For this review, take the finished solid that the model builds, in its own axes (mm). Face numbers are marked on the shaded views. Coordinates: 2 decimals unless noted, no trailing zeros. Loops run counter-clockwise (first coordinate to the right, second up) from the corner with the lowest first, then second, coordinate; pieces in that order, holes last. Notation, with made-up numbers: (-33, -35) - (23, -35) arc R13 cw to (23, -12) - close; hole circle Ø1 at (72.25, 76). An arc over 180 degrees is marked (long way). Use one line per item in the form item = value. Start each with the question number.
1. Add section C-C on z = 41. Give the boundary of the cut face in (x, y).
2. To check wall thickness, follow probe 1 along Y at (x, z) = (0, 23.25); probe 2 along Y at (x, z) = (0, 0.25); probe 3 along Z at (x, y) = (-8.5, -10.5). State the ranges of each line that lie inside material, in increasing order.
3. Add section A-A on z = 20.5. Give the boundary of the cut face in (x, y).
4. For pin 1 Ø1 at (x, z) = (3.5, 31.5) entering from +Y; pin 2 Ø2 at (x, z) = (-3.5, 41) entering from +Y; pin 3 Ø3 at (y, z) = (15, 38.5) entering from +X, all flat-tipped, find the tip position at first contact; note any pin that passes through.
5. Add section D-D on y = -11.25. Give the boundary of the cut face in (x, z).
6. Draft analysis for pull direction Y (two halves, no side actions). For the marked faces 1, 2 and 3, state which applies: +Y half, -Y half, draft (parallel to the pull), parting line (faces both ways), or undercut.
7. Add section B-B on x = 0. Give the boundary of the cut face in (y, z).
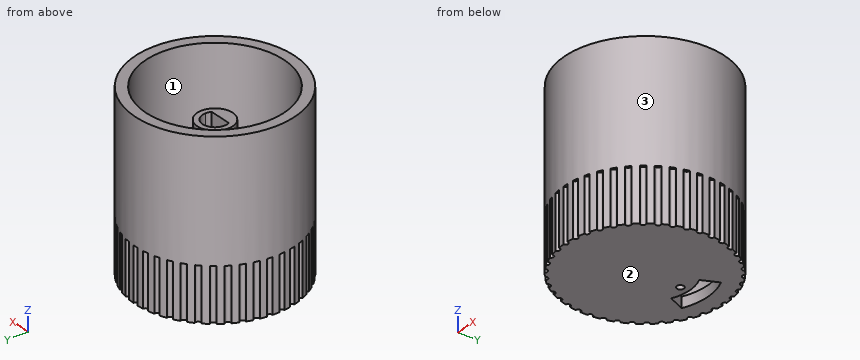
```python
from build123d import *

# Parameters (mm, degrees)
F10_R     = 22.5
F0_DEPTH  = 48.6
F1_T      = -3
F2_R      = 5
F3_DEPTH  = 37
F11_DEPTH = 30
F5_DEPTH  = 25
F13_R     = 1
F6_DEPTH  = 2
F7_R      = 1
F8_R      = 0.75
F9_DEPTH  = 15


with BuildPart() as f0:
    # F10 (on Top) → F0 (new body)
    with BuildSketch(Plane.XY):
        Circle(F10_R)
    extrude(amount=F0_DEPTH)

    # F1
    f1_openings = [f0.faces().sort_by_distance(p)[0] for p in [
        (0, 0, 48.6),
    ]]
    offset(amount=F1_T, openings=f1_openings)

    # F2 (on face) → F3 (join)
    with BuildSketch(Plane.XY.offset(3)):
        Circle(F2_R)
    extrude(amount=F3_DEPTH)

    # F4 (on face) → F11 (cut)
    with BuildSketch(Plane.XY.offset(40)):
        with BuildLine():
            ThreePointArc((3.1622776602, -1.5), (3.4145257219, -0.7687744108), (3.5, 0))
            ThreePointArc((3.5, 0), (-0.7687744108, 3.4145257219), (-3.1622776602, -1.5))
            Line((-3.1622776602, -1.5), (3.1622776602, -1.5))
        make_face()
    extrude(amount=-F11_DEPTH, mode=Mode.SUBTRACT)

    # F12 (on face) → F5 (cut)
    with BuildSketch(Plane.XY.offset(3)):
        with BuildLine():
            Line((5.1825942436, 11.3750040398), (7.255631941, 15.9250056558))
            Line((7.255631941, 15.9250056558), (-7.255631941, 15.9250056558))
            Line((-7.255631941, 15.9250056558), (-5.1825942436, 11.3750040398))
            ThreePointArc((-5.1825942436, 11.3750040398), (0, 12.5), (5.1825942436, 11.3750040398))
        make_face()
        with BuildLine():
            Line((-7.255631941, 15.9250056558), (7.255631941, 15.9250056558))
            ThreePointArc((7.255631941, 15.9250056558), (0, 17.5), (-7.255631941, 15.9250056558))
        make_face()
    extrude(amount=-F5_DEPTH, mode=Mode.SUBTRACT)

    # F13 (on face) → F6 (cut)
    with BuildSketch(Plane(origin=(0, 0, 0), x_dir=(1, 0, 0), z_dir=(0, 0, -1))):
        with Locations((0, -10)):
            Circle(F13_R)
    extrude(amount=-F6_DEPTH, mode=Mode.SUBTRACT)

    # F7
    f7_edges = [f0.edges().sort_by_distance(p)[0] for p in [
        (-1, 10, 2),
    ]]
    fillet(f7_edges, radius=F7_R)

    # F8 (on face) → F9 (cut)
    with BuildSketch(Plane(origin=(0, 0, 0), x_dir=(1, 0, 0), z_dir=(0, 0, -1))):
        with Locations((0, -22.5)):
            Circle(F8_R)
        with Locations((3.353450989, -22.2486935901)):
            Circle(F8_R)
        with Locations((6.6319914242, -21.5003881302)):
            Circle(F8_R)
        with Locations((9.7623841301, -20.2717995278)):
            Circle(F8_R)
        with Locations((12.6747013064, -18.5903724221)):
            Circle(F8_R)
        with Locations((15.3038865998, -16.4936671162)):
            Circle(F8_R)
        with Locations((17.5912083555, -14.0285205418)):
            Circle(F8_R)
        with Locations((19.4855715851, -11.25)):
            Circle(F8_R)
        with Locations((20.9446593445, -8.2201730482)):
            Circle(F8_R)
        with Locations((21.9358780241, -5.006721014)):
            Circle(F8_R)
        with Locations((22.4370854366, -1.6814271057)):
            Circle(F8_R)
        with Locations((22.4370854366, 1.6814271057)):
            Circle(F8_R)
        with Locations((21.9358780241, 5.006721014)):
            Circle(F8_R)
        with Locations((20.9446593445, 8.2201730482)):
            Circle(F8_R)
        with Locations((19.4855715851, 11.25)):
            Circle(F8_R)
        with Locations((17.5912083555, 14.0285205418)):
            Circle(F8_R)
        with Locations((15.3038865998, 16.4936671162)):
            Circle(F8_R)
        with Locations((12.6747013064, 18.5903724221)):
            Circle(F8_R)
        with Locations((9.7623841301, 20.2717995278)):
            Circle(F8_R)
        with Locations((6.6319914242, 21.5003881302)):
            Circle(F8_R)
        with Locations((3.353450989, 22.2486935901)):
            Circle(F8_R)
        with Locations((0, 22.5)):
            Circle(F8_R)
        with Locations((-3.353450989, 22.2486935901)):
            Circle(F8_R)
        with Locations((-6.6319914242, 21.5003881302)):
            Circle(F8_R)
        with Locations((-9.7623841301, 20.2717995278)):
            Circle(F8_R)
        with Locations((-12.6747013064, 18.5903724221)):
            Circle(F8_R)
        with Locations((-15.3038865998, 16.4936671162)):
            Circle(F8_R)
        with Locations((-17.5912083555, 14.0285205418)):
            Circle(F8_R)
        with Locations((-19.4855715851, 11.25)):
            Circle(F8_R)
        with Locations((-20.9446593445, 8.2201730482)):
            Circle(F8_R)
        with Locations((-21.9358780241, 5.006721014)):
            Circle(F8_R)
        with Locations((-22.4370854366, 1.6814271057)):
            Circle(F8_R)
        with Locations((-22.4370854366, -1.6814271057)):
            Circle(F8_R)
        with Locations((-21.9358780241, -5.006721014)):
            Circle(F8_R)
        with Locations((-20.9446593445, -8.2201730482)):
            Circle(F8_R)
        with Locations((-19.4855715851, -11.25)):
            Circle(F8_R)
        with Locations((-17.5912083555, -14.0285205418)):
            Circle(F8_R)
        with Locations((-15.3038865998, -16.4936671162)):
            Circle(F8_R)
        with Locations((-12.6747013064, -18.5903724221)):
            Circle(F8_R)
        with Locations((-9.7623841301, -20.2717995278)):
            Circle(F8_R)
        with Locations((-6.6319914242, -21.5003881302)):
            Circle(F8_R)
        with Locations((-3.353450989, -22.2486935901)):
            Circle(F8_R)
    extrude(amount=-F9_DEPTH, mode=Mode.SUBTRACT)


solid = f0.part
```
Conclusion:
q1.outline = circle Ø45 at (0, 0); hole circle Ø39 at (0, 0)
q2.probe_1 = -22.5 to -19.5, -5 to -1.5, 3.5 to 5, 19.5 to 22.5
q2.probe_2 = -21.75 to 9, 11 to 12.5, 17.5 to 21.75
q2.probe_3 = 0 to 3
q3.outline = circle Ø45 at (0, 0); circle Ø10 at (0, 0); hole circle Ø39 at (0, 0); hole (-3.16, -1.5) - (3.16, -1.5) arc R3.5 ccw (long way) to start
q4.pin_1 = 22.3
q4.pin_2 = 22.36
q4.pin_3 = 18
q5.outline = (-19.49, 15) - (-18.74, 15) - (-18.74, 0) - (18.74, 0) - (18.74, 15) - (19.49, 15) - (19.49, 48.6) - (15.93, 48.6) - (15.93, 3) - (-15.93, 3) - (-15.93, 48.6) - (-19.49, 48.6) - close
q6.face_1 = undercut
q6.face_2 = draft
q6.face_3 = parting line
q7.outline = (-22.5, 15) - (-21.75, 15) - (-21.75, 0) - (9, 0) - (9, 1) arc R1 cw to (11, 1) - (11, 0) - (12.5, 0) - (12.5, 3) - (5, 3) - (5, 40) - (3.5, 40) - (3.5, 10) - (-1.5, 10) - (-1.5, 40) - (-5, 40) - (-5, 3) - (-19.5, 3) - (-19.5, 48.6) - (-22.5, 48.6) - close; (17.5, 0) - (21.75, 0) - (21.75, 15) - (22.5, 15) - (22.5, 48.6) - (19.5, 48.6) - (19.5, 3) - (17.5, 3) - close
